Read the model definition and answer for the solid it produces. Units are mm, in the model's axes. A direction names the side the tool comes from. Give positions to 0.01 mm unless a question says otherwise; leave off trailing zeros. Order: outer loops, then holes, each group sorted by start corner. A loop starts at its lowest first (then second) coordinate and runs counter-clockwise, first axis right, second up.
Item 1: The mould has two halves that part along Y. Classify faces 1 (the face through (1.15, 0, 4)), 2 (the face through (-3, 3, 2.5)), 3 (the face through (6.466, 2.681, 6.792)), 4 (the face through (-1.75, 0.06, 3.55)): +Y half, -Y half, draft (parallel to the pull), parting line (faces both ways), or undercut.
Item 2: A cutting plane is placed at A-A (y = 0). Write down the section's boundary in (x, z), plus the area to 3 significant figures.
Item 3: A cutting plane is placed at C-C (z = 5.5). Write down the section's boundary in (x, y), plus the area to 3 significant figures.
Item 4: Find the intervals of material crossed by line 1 along X through (y, z) = (0, 5.25); line 2 along X through (y, z) = (0, 1.5); line 3 along Y through (x, z) = (0, 5.25), in increasing order.
Item 5: A cutting plane is placed at B-B (x = 0). Write down the section's boundary in (y, z).
Item 6: Which of the six approach directions +Z, -Z, +X, -X, +Y, -Y give full straight-line access (tool end or side, diameter ignored) to faces 5 (the face through (-0.867, 3.905, 1.268)), 6 (the face through (1.5, -0.1, 7)), 7 (the face through (-6, 0, 5))?
from build123d import *

# Parameters (mm, degrees)
F3_DEPTH = 7.001


with BuildPart() as f1:
    # F0 (on Front) → F1 (revolve)
    with BuildSketch(Plane.XZ):
        Polygon((0, 7), (0, 0), (4, 0), (4, 2.5), (7, 2.5), (7, 7), align=None)
    revolve(axis=Axis((0, 0, 3.5), (0, 0, -1)))

    # F2 (on face) → F3 (cut, through all)
    with BuildSketch(Plane.XY.offset(7)):
        with BuildLine():
            Line((1.15, -1.319091), (1.15, 1.319091))
            ThreePointArc((1.15, 1.319091), (-1.75, 0), (1.15, -1.319091))
        make_face()
    extrude(amount=-F3_DEPTH, mode=Mode.SUBTRACT)

    # F4 (on Front) → F5 (revolve, cut)
    with BuildSketch(Plane.XZ):
        Polygon((6, 4), (8.598076, 2.5), (8.598076, 7.5), (6, 6), align=None)
    revolve(axis=Axis((0, 0, 7), (0, 0, -1)), mode=Mode.SUBTRACT)


solid = f1.part
Response values:
1. face 1: undercut
1. face 2: draft
1. face 3: parting line
1. face 4: undercut
2. outline: (-7, 2.5) - (-4, 2.5) - (-4, 0) - (-1.75, 0) - (-1.75, 7) - (-7, 7) - (-7, 6.58) - (-6, 6) - (-6, 4) - (-7, 3.42) - close; (1.15, 0) - (4, 0) - (4, 2.5) - (7, 2.5) - (7, 3.42) - (6, 4) - (6, 6) - (7, 6.58) - (7, 7) - (1.15, 7) - close
2. area: 57.5 mm2
3. outline: circle Ø12 at (0, 0); hole (1.15, -1.32) - (1.15, 1.32) arc R1.75 ccw (long way) to start
3. area: 105 mm2
4. line 1: x = -6 to -1.75, 1.15 to 6
4. line 2: x = -4 to -1.75, 1.15 to 4
4. line 3: y = -6 to -1.75, 1.75 to 6
5. outline: (-7, 2.5) - (-4, 2.5) - (-4, 0) - (-1.75, 0) - (-1.75, 7) - (-7, 7) - (-7, 6.58) - (-6, 6) - (-6, 4) - (-7, 3.42) - close; (1.75, 0) - (4, 0) - (4, 2.5) - (7, 2.5) - (7, 3.42) - (6, 4) - (6, 6) - (7, 6.58) - (7, 7) - (1.75, 7) - close
6. face 5: -Z
6. face 6: +Z, +X, -X, +Y, -Y
6. face 7: none
